Can you work these out from the model? Positions are in its coordinate system, mm. A direction names the side the tool comes from. Give positions to 0.01 mm unless a question says otherwise; leave off trailing zeros. Order: outer loops, then holes, each group sorted by start corner. A loop starts at its lowest first (then second) coordinate and runs counter-clockwise, first axis right, second up. Notation, with made-up numbers: M 77,-37.5 L 98,-37.5 A18 ccw 98,-13.5 Z; hole C 31.5,-28 d10. An arc over 180 degrees is marked long. Use a Markdown table: item, result. Add a question column.
from build123d import *

# Parameters (mm, degrees)
SKETCH1_W               = 100
SKETCH1_H               = 120
BOSS_EXTRUDE1_DEPTH     = 8
SKETCH2_R               = 4.25
CUT_EXTRUDE1_DEPTH      = 8
MIRROR2_COPY_1_SKETCH_R = 4.25
MIRROR2_COPY_1_DEPTH    = 8
SKETCH3_R               = 16.25
CUT_EXTRUDE2_DEPTH      = 4
SKETCH4_R               = 29
BOSS_EXTRUDE2_DEPTH     = 50
SKETCH5_R               = 2.75
CUT_EXTRUDE3_DEPTH      = 70
SKETCH6_R               = 14
CUT_EXTRUDE4_DEPTH      = 31
SKETCH7_R               = 12.5
CUT_EXTRUDE5_DEPTH      = 61
SKETCH8_R               = 4.15
CUT_EXTRUDE6_DEPTH      = 6
CUT_EXTRUDE7_START      = -8.5
SKETCH9_R               = 14
CUT_EXTRUDE7_DEPTH      = 8.5


with BuildPart() as part:
    # Sketch1 → Boss-Extrude1 (new body)
    with BuildSketch(Plane.XY):
        Rectangle(SKETCH1_W, SKETCH1_H)
    extrude(amount=BOSS_EXTRUDE1_DEPTH)

    # Sketch2 → Cut-Extrude1 (cut)
    with BuildSketch(Plane.XY.offset(8)):
        with Locations((35, 45)):
            Circle(SKETCH2_R)
    cut_extrude1 = extrude(amount=-CUT_EXTRUDE1_DEPTH, mode=Mode.SUBTRACT)

    # Mirror1: Cut-Extrude1 across plane
    add(cut_extrude1.mirror(Plane(origin=(0, 0, 0), x_dir=(0, 0, 1), z_dir=(1, 0, 0))), mode=Mode.SUBTRACT)

    # Mirror2: Cut-Extrude1 across plane
    add(cut_extrude1.mirror(Plane.ZX), mode=Mode.SUBTRACT)

    # Mirror2 copy 1 sketch → Mirror2 copy 1 (cut)
    with BuildSketch(Plane(origin=(0, 0, 8), x_dir=(-1, 0, 0), z_dir=(0, 0, 1))):
        with Locations((35, 45)):
            Circle(MIRROR2_COPY_1_SKETCH_R)
    extrude(amount=-MIRROR2_COPY_1_DEPTH, mode=Mode.SUBTRACT)

    # Sketch3 → Cut-Extrude2 (cut)
    with BuildSketch(Plane.XY.offset(8)):
        Circle(SKETCH3_R)
    extrude(amount=-CUT_EXTRUDE2_DEPTH, mode=Mode.SUBTRACT)

    # Sketch4 → Boss-Extrude2 (add)
    with BuildSketch(Plane(origin=(0, 0, 0), x_dir=(-1, 0, 0), z_dir=(0, 0, -1))):
        Circle(SKETCH4_R)
    extrude(amount=BOSS_EXTRUDE2_DEPTH)

    # Sketch5 → Cut-Extrude3 (cut)
    with BuildSketch(Plane.XY.offset(8)):
        with Locations((0, 23)):
            Circle(SKETCH5_R)
        with Locations((23, 0)):
            Circle(SKETCH5_R)
        with Locations((0, -23)):
            Circle(SKETCH5_R)
        with Locations((-23, 0)):
            Circle(SKETCH5_R)
    extrude(amount=-CUT_EXTRUDE3_DEPTH, mode=Mode.SUBTRACT)

    # Sketch6 → Cut-Extrude4 (cut)
    with BuildSketch(Plane.XY.offset(4)):
        Circle(SKETCH6_R)
    extrude(amount=-CUT_EXTRUDE4_DEPTH, mode=Mode.SUBTRACT)

    # Sketch7 → Cut-Extrude5 (cut)
    with BuildSketch(Plane.XY.offset(-27)):
        Circle(SKETCH7_R)
    extrude(amount=-CUT_EXTRUDE5_DEPTH, mode=Mode.SUBTRACT)

    # Sketch8 → Cut-Extrude6 (cut)
    with BuildSketch(Plane(origin=(0, 0, -50), x_dir=(-1, 0, 0), z_dir=(0, 0, -1))):
        with Locations((0, 23)):
            Circle(SKETCH8_R)
        with Locations((23, 0)):
            Circle(SKETCH8_R)
        with Locations((0, -23)):
            Circle(SKETCH8_R)
        with Locations((-23, 0)):
            Circle(SKETCH8_R)
    extrude(amount=-CUT_EXTRUDE6_DEPTH, mode=Mode.SUBTRACT)

    # Sketch9 → Cut-Extrude7 (cut)
    with BuildSketch(Plane(origin=(0, 0, -50), x_dir=(-1, 0, 0), z_dir=(0, 0, -1)).offset(CUT_EXTRUDE7_START)):
        with Locations(Location((0, 0, 0), (0, 0, 180))):
            Circle(SKETCH9_R)
    extrude(amount=CUT_EXTRUDE7_DEPTH, mode=Mode.SUBTRACT)


solid = part.part
1. We'd pull the mould along X, two halves only. Please class faces 4 (the face through (-0.358, 25.727, -17.636)), 5 (the face through (-50, -1, 4)), 6 (the face through (-18.854, 0.182, -47.042)), 7 (the face through (-13.38, -25.73, -24.65)): +X half, -X half, draft (parallel to the pull), parting line (faces both ways), or undercut.
2. On a 3-axis mill with a long thin cutter (end or side, diameter ignored), from which of +Z, -Z, +X, -X, +Y, -Y can I reach the whole of each face in a straight line? I mean faces 1 (the face through (50, -1, 4)), 2 (the face through (12.932, -5.362, -11.283)), 3 (the face through (12.932, 5.362, -45.69)). Say none if no direction works.
3. I need wall thicknesses on L1, parallel to Y at x = 0, z = -22; L2, parallel to Y at x = 35, z = 2; L3, parallel to Y at x = 0, z = -46.25. Which ranges of each line are inside material? Lowest first, please. Write a range as [from, to].
4. If we section it at C-C, the plane z = 2: State how many separate pieces and enclosed holes the cut face has, then the cut area to 3 significant figures.
5. Will these pins go through, and if not, where does the flat tip stop? pin 1 (4 mm diameter, centred on x = -8, z = -22, fed in from +Y); pin 2 (1 mm diameter, centred on x = 18, z = -23, fed in from +Y); pin 3 (12 mm diameter, centred on x = 36.5, y = -47, fed in from -Z); pin 4 (3.5 mm diameter, centred on x = -23, y = 0, fed in from +Z).
6. If we section it at D-D, the plane z = -39.5: List the corners of the cut face in (x, y) for me, then the cut area to 3 significant figures.
7. If we section it at B-B, the plane x = 35: List the corners of the cut face in (y, z) for me, then the cut area to 3 significant figures.
8. If we section it at A-A, the plane y = -45: List the corners of the cut face in (x, z) for me.
Geometry results:
| question | item | result |
|---|---|---|
| 1 | face 4 | undercut |
| 1 | face 5 | -X half |
| 1 | face 6 | undercut |
| 1 | face 7 | parting line |
| 2 | face 1 | +Z, -Z, +X, +Y, -Y |
| 2 | face 2 | +Z |
| 2 | face 3 | -Z |
| 3 | L1 | y = [-29, -25.75], [-20.25, -14], [14, 20.25], [25.75, 29] |
| 3 | L2 | y = [-60, -49.25], [-40.75, 40.75], [49.25, 60] |
| 3 | L3 | y = [-29, -27.15], [-18.85, -14], [14, 18.85], [27.15, 29] |
| 4 | separate pieces | 1 |
| 4 | enclosed holes | 9 |
| 4 | area | 11,100 mm^2 |
| 5 | pin 1 | stops at y = 28.37 |
| 5 | pin 2 | stops at y = 23.12 |
| 5 | pin 3 | stops at z = 0 |
| 5 | pin 4 | passes through |
| 6 | outline | C 0,0 d58; hole C -23,0 d5.5; hole C 0,0 d25; hole C 0,-23 d5.5; hole C 0,23 d5.5; hole C 23,0 d5.5 |
| 6 | area | 2,060 mm^2 |
| 7 | outline | M -60,0 L -49.25,0 L -49.25,8 L -60,8 Z; M -40.75,0 L 40.75,0 L 40.75,8 L -40.75,8 Z; M 49.25,0 L 60,0 L 60,8 L 49.25,8 Z |
| 7 | area | 824 mm^2 |
| 8 | outline | M -50,0 L -39.25,0 L -39.25,8 L -50,8 Z; M -30.75,0 L 30.75,0 L 30.75,8 L -30.75,8 Z; M 39.25,0 L 50,0 L 50,8 L 39.25,8 Z |
